Can you work these out from the model? Positions are in its coordinate system, mm. A direction names the side the tool comes from. Round coordinates to 2 decimals unless told otherwise and drop trailing zeros. Order: outer loops, then holes, each group sorted by start corner. A loop starts at its lowest first (then second) coordinate and runs counter-clockwise, first axis right, second up. Notation, with made-up numbers: M 55.5,65.25 L 72.5,65.25 A10 ccw 72.5,78.25 Z; hole C 72.5,26 d2. An arc over 180 degrees is marked long. Answer as a JSON object with one key per item and string values. Group by question number.
```python
from build123d import *

# Parameters (mm, degrees)
EXTRUDE1_DEPTH = 25.4


with BuildPart() as part:
    # Sketch2 → Extrude1 (new body)
    with BuildSketch(Plane.XY):
        with BuildLine():
            Line((0, 0), (75.929788313, 0))
            Line((75.929788313, 0), (75.929788313, 68.608572188))
            ThreePointArc((75.929788313, 68.608572188), (76.25000769, 71.442479692), (77.194517721, 74.133478204))
            Line((77.194517721, 74.133478204), (114.663486186, 151.685529213))
            Line((114.663486186, 151.685529213), (87.189584206, 199.877455637))
            Line((87.189584206, 199.877455637), (0, 199.877455637))
            Line((0, 199.877455637), (0, 0))
        make_face()
    extrude(amount=-EXTRUDE1_DEPTH)


solid = part.part
```
1) For pin 1 (2 mm diameter, centred on y = 40.5, z = -7.5, fed in from +X), with a flat end and sliding along its axis, tell me the tip position at first contact or that it passes through.
2) If we section it at B-B on x = 82: Write out the boundary of the cut face in (y, z).
3) If we section it at C-C on y = 155.5: Write out the boundary of the cut face in (x, z).
4) I need wall thicknesses on line 1 along X through (y, z) = (27, -20.75); line 2 along X through (y, z) = (135, -16.75); line 3 along Y through (x, z) = (103.5, -9.25). Which ranges of each line are inside material? Lowest first, please.
5) Which directions (+Z, -Z, +X, -X, +Y, -Y) give clear straight access to the entire face, cutting with the end or side of a thin tool? Please do faces 1 (the face through (44, 101, -25.4)), 2 (the face through (75.93, 34, -13)).
6) If we section it at A-A on z = -11.5: Write out the boundary of the cut face in (x, y), plus the area to 3 significant figures.
Findings:
{
 "1": {"pin 1": "stops at x = 75.93"},
 "2": {"outline": "M 84.08,-25.4 L 199.88,-25.4 L 199.88,0 L 84.08,0 Z"},
 "3": {"outline": "M 0,-25.4 L 112.49,-25.4 L 112.49,0 L 0,0 Z"},
 "4": {"line 1": "x = 0 to 75.93", "line 2": "x = 0 to 106.6", "line 3": "y = 128.58 to 171.27"},
 "5": {"face 1": "-Z, +X, -X, +Y, -Y", "face 2": "+Z, -Z, +X, -Y"},
 "6": {"outline": "M 0,0 L 75.93,0 L 75.93,68.61 A12.7 cw 77.19,74.13 L 114.66,151.69 L 87.19,199.88 L 0,199.88 Z", "area": "17,900 mm^2"}
}
